Build history of the part. All positions in model axes, mm. Coordinates: 2 decimals unless noted, no trailing zeros. Loops run counter-clockwise (first coordinate to the right, second up) from the corner with the lowest first, then second, coordinate; pieces in that order, holes last.
Item 1: Cut at A-A (x = 29). List the corners of the cut face in (y, z), and give its area (3 significant figures).
Item 2: Drill centre lines: line 1 along Z through (x, y) = (71, 25.75); line 2 along Y through (x, z) = (27.5, 5.5). Where is each one in solid material? Low to high.
Item 3: Flat gauge pins, fed straight in: pin 1 (3 mm diameter, centred on x = 51.5, y = 26, fed in from -Z); pin 2 (3.5 mm diameter, centred on y = 25.75, z = 5.5, fed in from -X); pin 3 (2 mm diameter, centred on x = 48, y = 26.5, fed in from +Z); pin 4 (2 mm diameter, centred on x = 35, y = 26.5, fed in from -Z). Where does each tip first touch, or does it go through?
Item 4: Cut at B-B (z = -5.5). List the corners of the cut face in (x, y).
from build123d import *

# Parameters (mm, degrees)
EXTRUDE_1_DEPTH             = 90
SKETCH_2_W                  = 90
SKETCH_2_H                  = 17.75
EXTRUDE_2_DEPTH             = 8.2
SKETCH_3_W                  = 90
SKETCH_3_H                  = 50.95
EXTRUDE_3_DEPTH             = 8.2
SKETCH_4_W                  = 3.95
SKETCH_4_H                  = 29.5
CUT_EXTRUDE_1_DEPTH         = 96.44153315
SKETCH_5_W                  = 3.95
SKETCH_5_H                  = 6.2
CUT_EXTRUDE_2_DEPTH         = 96.44153315
SKETCH_6_W                  = 2.25
SKETCH_6_H                  = 3.95
CUT_EXTRUDE_3_DEPTH         = 96.44153315
SKETCH_7_W                  = 4.5
SKETCH_7_H                  = 3.95
CUT_EXTRUDE_4_DEPTH         = 96.44153315
SKETCH_8_W                  = 2.25
SKETCH_8_H                  = 3.95
CUT_EXTRUDE_5_DEPTH         = 96.44153315
SKETCH_9_W                  = 3.95
SKETCH_9_H                  = 2.25
CUT_EXTRUDE_6_DEPTH         = 96.44153315
SKETCH_10_W                 = 20.2
SKETCH_10_H                 = 45.2
CUT_EXTRUDE_7_DEPTH         = 86
HOLE_WIZARD_2_5_2_5_1_D     = 2.5
HOLE_WIZARD_4_5_4_5_1_D     = 4.5
HOLE_WIZARD_8_3_8_3_1_D     = 8.3
HOLE_WIZARD_8_3_8_3_1_DEPTH = 3.2
FILLET_1_R                  = 2
FILLET_2_R                  = 2
EXTRUDE_START               = -90
SKETCH_17_R                 = 1.25
EXTRUDE_4_DEPTH             = 90
CUT_EXTRUDE_START           = -100
SKETCH_18_R                 = 4.15
CUT_EXTRUDE_8_DEPTH         = 100
CUT_EXTRUDE_9_DEPTH         = 130
SKETCH_20_W                 = 90
SKETCH_20_H                 = 22.108571968
EXTRUDE_5_DEPTH             = 2


with BuildPart() as part:
    # Эскиз1 → Бобышка-Вытянуть1 (new body)
    with BuildSketch(Plane(origin=(90, 0, 0), x_dir=(0, 0, -1), z_dir=(1, 0, 0))):
        with BuildLine():
            Line((6.75, -24.093761792), (6.75, 19.25))
            Line((6.75, 19.25), (-11.593761792, 19.25))
            ThreePointArc((-11.593761792, 19.25), (-15.325, 18), (-11.593761792, 16.75))
            Line((-11.593761792, 16.75), (-11, 16.75))
            Line((-11, 16.75), (-11, -16.75))
            Line((-11, -16.75), (-11.593761792, -16.75))
            ThreePointArc((-11.593761792, -16.75), (-15.325, -18), (-11.593761792, -19.25))
            Line((-11.593761792, -19.25), (-11, -19.25))
            Line((-11, -19.25), (-11, -23.5))
            Line((-11, -23.5), (-6.75, -23.5))
            Line((-6.75, -23.5), (-6.75, -24.093761792))
            ThreePointArc((-6.75, -24.093761792), (-5.5, -27.825), (-4.25, -24.093761792))
            Line((-4.25, -24.093761792), (-4.25, -23.5))
            Line((-4.25, -23.5), (4.25, -23.5))
            Line((4.25, -23.5), (4.25, -24.093761792))
            ThreePointArc((4.25, -24.093761792), (5.5, -27.825), (6.75, -24.093761792))
        make_face()
    extrude(amount=-EXTRUDE_1_DEPTH)

    # Эскиз2 → Бобышка-Вытянуть2 (add)
    with BuildSketch(Plane(origin=(0, 19.25, 0), x_dir=(-1, 0, 0), z_dir=(0, 1, 0))):
        with Locations((-45, 2.125)):
            Rectangle(SKETCH_2_W, SKETCH_2_H)
    extrude(amount=EXTRUDE_2_DEPTH)

    # Эскиз3 → Бобышка-Вытянуть3 (add)
    with BuildSketch(Plane(origin=(0, 0, -6.75), x_dir=(-1, 0, 0), z_dir=(0, 0, -1))):
        with Locations((-45, 1.975)):
            Rectangle(SKETCH_3_W, SKETCH_3_H)
    extrude(amount=EXTRUDE_3_DEPTH)

    # Эскиз4 → Вырез-Вытянуть1 (cut, through all)
    with BuildSketch(Plane.ZY):
        with Locations((-12.975, 0)):
            Rectangle(SKETCH_4_W, SKETCH_4_H)
    extrude(amount=-CUT_EXTRUDE_1_DEPTH, mode=Mode.SUBTRACT)

    # Эскиз5 → Вырез-Вытянуть2 (cut, through all)
    with BuildSketch(Plane.ZY):
        with Locations((-12.975, 24.35)):
            Rectangle(SKETCH_5_W, SKETCH_5_H)
    extrude(amount=-CUT_EXTRUDE_2_DEPTH, mode=Mode.SUBTRACT)

    # Эскиз6 → Вырез-Вытянуть3 (cut, through all)
    with BuildSketch(Plane.ZY):
        with Locations((-9.875, 25.475)):
            Rectangle(SKETCH_6_W, SKETCH_6_H)
    extrude(amount=-CUT_EXTRUDE_3_DEPTH, mode=Mode.SUBTRACT)

    # Эскиз7 → Вырез-Вытянуть4 (cut, through all)
    with BuildSketch(Plane.ZY):
        with Locations((0, 25.475)):
            Rectangle(SKETCH_7_W, SKETCH_7_H)
    extrude(amount=-CUT_EXTRUDE_4_DEPTH, mode=Mode.SUBTRACT)

    # Эскиз8 → Вырез-Вытянуть5 (cut, through all)
    with BuildSketch(Plane.ZY):
        with Locations((9.875, 25.475)):
            Rectangle(SKETCH_8_W, SKETCH_8_H)
    extrude(amount=-CUT_EXTRUDE_5_DEPTH, mode=Mode.SUBTRACT)

    # Эскиз9 → Вырез-Вытянуть6 (cut, through all)
    with BuildSketch(Plane.ZY):
        with Locations((-12.975, -22.375)):
            Rectangle(SKETCH_9_W, SKETCH_9_H)
    extrude(amount=-CUT_EXTRUDE_6_DEPTH, mode=Mode.SUBTRACT)

    # Эскиз10 → Вырез-Вытянуть7 (cut)
    with BuildSketch(Plane(origin=(90, 0, 0), x_dir=(0, 0, -1), z_dir=(1, 0, 0))):
        Rectangle(SKETCH_10_W, SKETCH_10_H)
    extrude(amount=-CUT_EXTRUDE_7_DEPTH, mode=Mode.SUBTRACT)

    # Диаметр отверстия Ø2.5 (2.5)1 (through all)
    with Locations(Plane(origin=(90, 0, 0), x_dir=(0, 0, -1), z_dir=(1, 0, 0))):
        with Locations((5.5, -25.75), (-13.25, -18), (-5.5, -25.75), (-13.25, 18)):
            Hole(HOLE_WIZARD_2_5_2_5_1_D / 2)

    # Диаметр отверстия Ø4.5 (4.5)1 (through all)
    with Locations(Plane.ZY):
        with Locations((-13.25, -18), (-13.25, 18), (-5.5, 25.75), (5.5, 25.75)):
            Hole(HOLE_WIZARD_4_5_4_5_1_D / 2)

    # Диаметр отверстия Ø8.3 (8.3)1
    with Locations(Plane.ZY):
        with Locations((0, 0)):
            Hole(HOLE_WIZARD_8_3_8_3_1_D / 2, depth=HOLE_WIZARD_8_3_8_3_1_DEPTH)

    # Скругление1
    fillet_1_edges = [part.edges().sort_by_distance(p)[0] for p in [
        (45, 23.5, 8.75),
    ]]
    fillet(fillet_1_edges, radius=FILLET_1_R)

    # Скругление2
    fillet_2_edges = [part.edges().sort_by_distance(p)[0] for p in [
        (45, 23.5, -8.75),
        (45, 23.5, 2.25),
        (45, 23.5, -2.25),
        (45, -21.25, -11),
        (4, 0, -10.1),
        (4, -22.6, 0),
        (4, 0, 10.1),
        (4, 22.6, 0),
        (45, 14.75, -11),
        (45, -14.75, -11),
        (45, 21.25, -11),
    ]]
    fillet(fillet_2_edges, radius=FILLET_2_R)

    # Эскиз17 → Бобышка-Вытянуть4 (add)
    with BuildSketch(Plane(origin=(90, 0, 0), x_dir=(0, 0, -1), z_dir=(1, 0, 0)).offset(EXTRUDE_START)):
        with Locations((5.5, -25.75)):
            Circle(SKETCH_17_R)
        with Locations((-5.5, -25.75)):
            Circle(SKETCH_17_R)
        with Locations((-13.25, -18)):
            Circle(SKETCH_17_R)
        with Locations((-13.25, 18)):
            Circle(SKETCH_17_R)
    extrude(amount=EXTRUDE_4_DEPTH)

    # Эскиз18 → Вырез-Вытянуть8 (cut)
    with BuildSketch(Plane.ZY.offset(CUT_EXTRUDE_START)):
        Circle(SKETCH_18_R)
    extrude(amount=CUT_EXTRUDE_8_DEPTH, mode=Mode.SUBTRACT)

    # Эскиз19 → Вырез-Вытянуть9 (cut)
    with BuildSketch(Plane(origin=(90, 0, 0), x_dir=(0, 0, -1), z_dir=(1, 0, 0))):
        Polygon((10.1, 22.6), (-10.1, 22.6), (-23.41122638, 22.6), (-23.41122638, -34.175581762), (22.796675715, -34.175581762), (22.796675715, 22.6), align=None)
    extrude(amount=-CUT_EXTRUDE_9_DEPTH, mode=Mode.SUBTRACT)

    # Эскиз20 → Бобышка-Вытянуть5 (add)
    with BuildSketch(Plane.XZ.offset(-22.6)):
        with Locations((45, -0.054285984)):
            Rectangle(SKETCH_20_W, SKETCH_20_H)
    extrude(amount=EXTRUDE_5_DEPTH)


solid = part.part
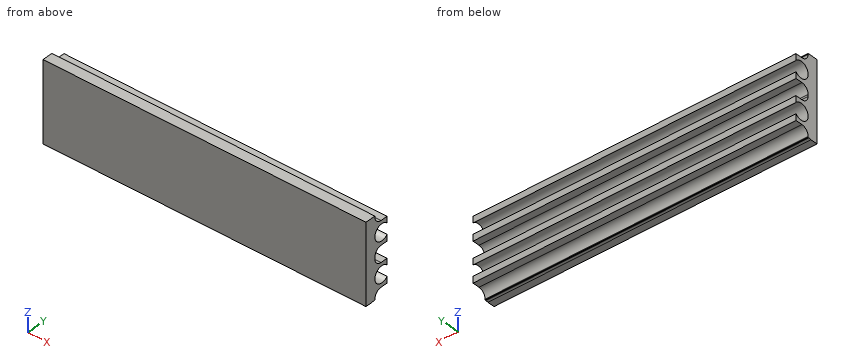
Filled sheet:
1. outline: (20.6, -11.11) - (22.6, -11.11) arc R2 cw to (23.25, -11) - (23.5, -11) - (23.5, -10.75) arc R2 cw to (25.5, -8.75) - (27.45, -8.75) - (27.45, -6.97) arc R2.25 cw (long way) to (27.45, -4.03) - (27.45, -2.25) - (25.5, -2.25) arc R2 cw to (23.5, -0.25) - (23.5, 0.25) arc R2 cw to (25.5, 2.25) - (27.45, 2.25) - (27.45, 4.03) arc R2.25 cw (long way) to (27.45, 6.97) - (27.45, 8.75) - (25.5, 8.75) arc R2 cw to (23.5, 10.75) - (23.5, 11) - (20.6, 11) - close
1. area: 89.2 mm2
2. line 1: z = -8.75 to -7.75, -3.25 to -2.25, 2.25 to 3.25, 7.75 to 8.75
2. line 2: y = 20.6 to 23.5
3. pin 1: stops at z = -9.02
3. pin 2: passes through
3. pin 3: stops at z = 8.75
3. pin 4: stops at z = -8.75
4. outline: (0, 20.6) - (90, 20.6) - (90, 23.5) - (0, 23.5) - close
